Part model, mm, in its own coordinate system. A direction names the side the tool comes from. Give positions to 0.01 mm unless a question says otherwise; leave off trailing zeros. Write each loop counter-clockwise with the first axis right and the second up, starting at its lowest first coordinate (ties: lowest second). Pieces come first, ordered by that corner, then holes. Notation, with made-up numbers: (43.25, 40.25) - (97.25, 40.25) arc R35 cw to (97.25, 75.25) - close; hole circle Ø2 at (-12.5, 56.25). An arc over 180 degrees is marked (long way). Answer in a Markdown table with one row per item. Add a question column.
1. Band-saw the part on B-B on y = -21.5. Write the cut outline in (x, z) (3 decimals).
2. Probe line 1 along Z through (x, y) = (27.65, 21.5) (3 decimals); line 2 along Z through (x, y) = (24.6, 21.5); line 3 along X through (y, z) = (-4, 6). List the from-to ranges inside material, lowest first.
3. Drop flat-ended pins along their axis: pin 1 Ø3 at (y, z) = (-21.5, 6) entering from +X; pin 2 Ø12 at (x, y) = (-13.5, -1.5) entering from +Z; pin 3 Ø3 at (x, y) = (0.5, 2) entering from -Z. Give the stop position or say it passes through.
4. Pull direction Z, two halves, no side cores. Call faces 4 (the flat face through (0, 30, 11)), 5 (the flat face through (-3, 0, 8)), 6 (the cylindrical face through (28.27, 18.43, 4.64)): released by +Z, released by -Z, zero draft, split by the parting line, or undercut.
5. Band-saw the part on A-A on z = 4.5. Write the cut outline in (x, y) (3 decimals).
6. Band-saw the part on D-D on x = 12.5. Write the cut outline in (y, z).
7. Which spindle directions (+Z, -Z, +X, -X, +Y, -Y) get a long thin tool onto all of the face, cutting with end or side? Do faces 1 (the flat face through (3, 0, 14)), 2 (the flat face through (26.5, 21, 2)), 3 (the flat face through (24, 0, 4)). Say none if no direction does.
8. Band-saw the part on C-C on y = -0.5. Write the cut outline in (x, z).
```python
from build123d import *

# Parameters (mm, degrees)
F0_W     = 60
F0_H     = 60
F1_DEPTH = 22
F2_W     = 65.936946
F2_H     = 73.230896
F3_DEPTH = 8
F4_W     = 66.143565
F4_H     = 69.968968
F5_DEPTH = 8
F6_R     = 2
F7_DEPTH = 8
F8_R     = 3.075
F9_DEPTH = 3.5


with BuildPart() as f1:
    # F0 (on Top) → F1 (new body)
    with BuildSketch(Plane.XY):
        Rectangle(F0_W, F0_H)
    extrude(amount=F1_DEPTH)

    # F2 (on face) → F3 (cut)
    with BuildSketch(Plane.XY.offset(22)):
        with Locations((8.968473, 0)):
            Rectangle(F2_W, F2_H)
    extrude(amount=-F3_DEPTH, mode=Mode.SUBTRACT)

    # F4 (on face) → F5 (cut)
    with BuildSketch(Plane(origin=(0, 0, 0), x_dir=(1, 0, 0), z_dir=(0, 0, -1))):
        with Locations((-9.071782, 0)):
            Rectangle(F4_W, F4_H)
    extrude(amount=-F5_DEPTH, mode=Mode.SUBTRACT)

    # F6 (on face) → F7 (cut)
    with BuildSketch(Plane.YZ.offset(30)):
        with Locations((21.5, 4.5)):
            Circle(F6_R)
        with Locations((-21.5, 4.5)):
            Circle(F6_R)
    extrude(amount=-F7_DEPTH, mode=Mode.SUBTRACT)

    # F8 (on face) → F9 (cut)
    with BuildSketch(Plane.YZ.offset(30)):
        with Locations((-21.5, 4.5)):
            Circle(F8_R)
        with Locations((21.5, 4.5)):
            Circle(F8_R)
    extrude(amount=-F9_DEPTH, mode=Mode.SUBTRACT)


solid = f1.part
```
Values:
| question | item | result |
|---|---|---|
| 1 | outline | (-30, 8) - (24, 8) - (24, 6.5) - (26.5, 6.5) - (26.5, 7.575) - (30, 7.575) - (30, 14) - (-24, 14) - (-24, 22) - (-30, 22) - close; (24, 0) - (30, 0) - (30, 1.425) - (26.5, 1.425) - (26.5, 2.5) - (24, 2.5) - close |
| 2 | line 1 | z = 0 to 1.425, 7.575 to 14 |
| 2 | line 2 | z = 0 to 2.5, 6.5 to 14 |
| 2 | line 3 | x = 24 to 30 |
| 3 | pin 1 | stops at x = 26.5 |
| 3 | pin 2 | stops at z = 14 |
| 3 | pin 3 | stops at z = 8 |
| 4 | face 4 | zero draft |
| 4 | face 5 | released by -Z |
| 4 | face 6 | undercut |
| 5 | outline | (24, -30) - (30, -30) - (30, -24.575) - (26.5, -24.575) - (26.5, -23.5) - (24, -23.5) - close; (24, -19.5) - (26.5, -19.5) - (26.5, -18.425) - (30, -18.425) - (30, 18.425) - (26.5, 18.425) - (26.5, 19.5) - (24, 19.5) - close; (24, 23.5) - (26.5, 23.5) - (26.5, 24.575) - (30, 24.575) - (30, 30) - (24, 30) - close |
| 6 | outline | (-30, 8) - (30, 8) - (30, 14) - (-30, 14) - close |
| 7 | face 1 | +Z, +X, +Y, -Y |
| 7 | face 2 | +X |
| 7 | face 3 | -Z, -X, +Y, -Y |
| 8 | outline | (-30, 8) - (24, 8) - (24, 0) - (30, 0) - (30, 14) - (-24, 14) - (-24, 22) - (-30, 22) - close |
